Geometry check sheet. Reference: the model listing, model coordinates, mm. A direction names the side the tool comes from. Round coordinates to 2 decimals unless told otherwise and drop trailing zeros. Write each loop counter-clockwise with the first axis right and the second up, starting at its lowest first coordinate (ties: lowest second). Pieces come first, ordered by that corner, then holes. Notation, with made-up numbers: (21, 65.25) - (40, 65.25) arc R22 ccw to (40, 94.25) - close; hole circle Ø11 at (36, 7.5). An arc over 180 degrees is marked (long way). Return JSON: item names as keys, results as strings.
```python
from build123d import *

# Parameters (mm, degrees)
BOSS_EXTRUDE1_DEPTH = 1.5875
FILLET1_R           = 3.81
FILLET2_R           = 1.5875
SKETCH8_R           = 2.25
CUT_EXTRUDE1_DEPTH  = 3.175


with BuildPart() as part:
    # Sketch1 → Boss-Extrude1 (new body)
    with BuildSketch(Plane(origin=(0, 0, 0), x_dir=(1, 0, 0), z_dir=(0, 1, 0))):
        with BuildLine():
            Line((-247.50833587, -59.933994147), (-240.439659658, -89.034683934))
            add(Edge.make_bspline(
                [(-240.439659658, -89.034683934), (-242.558073639, -80.3134883), (-236.877012866, -74.608932784), (-230.317813562, -73.452368974), (-229.725859184, -73.347991446), (-229.113793878, -73.283589588), (-228.485146838, -73.26562397)],
                knots=[0.241984005, 0.241984005, 0.241984005, 0.241984005, 0.5, 0.5, 0.5, 0.533893072, 0.533893072, 0.533893072, 0.533893072], degree=3, weights=[0.500514049, 0.489483356, 0.655978673, 1, 0.954809238, 0.912681783, 0.873617635]))
            Line((-228.485146838, -73.26562397), (-234.80833587, -47.233994147))
            Line((-234.80833587, -47.233994147), (-234.80833587, -12.308994147))
            ThreePointArc((-234.80833587, -12.308994147), (-235.738271839, -10.063930117), (-237.98333587, -9.133994147))
            Line((-237.98333587, -9.133994147), (-244.33333587, -9.133994147))
            ThreePointArc((-244.33333587, -9.133994147), (-246.5783999, -10.063930117), (-247.50833587, -12.308994147))
            Line((-247.50833587, -12.308994147), (-247.50833587, -59.933994147))
        make_face()
    extrude(amount=BOSS_EXTRUDE1_DEPTH)

    # Fillet1
    fillet1_edges = [part.edges().sort_by_distance(p)[0] for p in [
        (-228.485146838, 0.79375, 73.26562397),
    ]]
    fillet(fillet1_edges, radius=FILLET1_R)

    # Fillet2
    fillet2_edges = [part.edges().sort_by_distance(p)[0] for p in [
        (-240.439659658, 0.79375, 89.034683934),
    ]]
    fillet(fillet2_edges, radius=FILLET2_R)

    # Sketch8 → Cut-Extrude1 (cut)
    with BuildSketch(Plane(origin=(0, 1.5875, 0), x_dir=(1, 0, 0), z_dir=(0, 1, 0))):
        with Locations(Location((-241.15833587, -21.833994147, 0), (0, 0, 270))):
            Circle(SKETCH8_R)
        with Locations(Location((-241.15833587, -47.233994147, 0), (0, 0, 270))):
            Circle(SKETCH8_R)
    extrude(amount=-CUT_EXTRUDE1_DEPTH, mode=Mode.SUBTRACT)


solid = part.part
```
(1) Material ranges on line 1 along Z through (x, y) = (-241, 1.3); line 2 along Z through (x, y) = (-242.25, 0.2); line 3 along X through (y, z) = (0.75, 46), recorded low to high. Write a range as [from, to].
Response values:
{"line 1": "z = [9.13, 19.59], [24.08, 44.99], [49.48, 81.48]", "line 2": "z = [9.13, 19.87], [23.8, 45.27], [49.2, 80.9]", "line 3": "x = [-247.51, -243.04], [-239.28, -234.81]"}
(2) Release check for a two-part mould opening along X. For faces 3 (the face through (-245.074, 0.783, 69.957)), 4 (the face through (-239.26, 0.8, 48.44)), 5 (the face through (-240.6, 1.588, 44.8)) record: pulls with the +X half, pulls with the -X half, needs draft (parallel to the pull), parting line crosses it, or undercut.
Response values:
{"face 3": "pulls with the -X half", "face 4": "undercut", "face 5": "needs draft"}
(3) Section check C-C, the plane y = 0.95. Give the number of separate pieces and of enclosed holes in the cut face, plus the area to 3 significant figures.
Response values:
{"separate pieces": "1", "enclosed holes": "2", "area": "889 mm^2"}
(4) Section check B-B, the plane x = -245. Enter the section's corners in (y, z).
Response values:
{"outline": "(0, 9.2) - (1.59, 9.2) - (1.59, 70.26) - (0, 70.26) - close"}
(5) Section check D-D, the plane z = 66. Enter the section's corners in (x, y), plus the area to 3 significant figures.
Response values:
{"outline": "(-246.03, 0) - (-230.25, 0) - (-230.25, 1.59) - (-246.03, 1.59) - close", "area": "25.1 mm^2"}
(6) Access from +Z, -Z, +X, -X, +Y, -Y to the whole of each face (thin tool, end or side, straight path). Record for faces 1 (the face through (-234.808, 1, 30)), 2 (the face through (-240.6, 0, 44.8)).
Response values:
{"face 1": "-Z, +X, +Y, -Y", "face 2": "+Z, -Z, +X, -X, -Y"}
(7) Section check A-A, the plane z = 48. Enter the section's corners in (x, y).
Response values:
{"outline": "(-247.51, 0) - (-243.27, 0) - (-243.27, 1.59) - (-247.51, 1.59) - close; (-239.04, 0) - (-234.62, 0) - (-234.62, 1.59) - (-239.04, 1.59) - close"}
